Check sheet for the modelled part. Datum: model origin and axes. Units: mm. Face numbers are marked on the shaded views. A direction names the side the tool comes from. Give positions to 0.01 mm unless a question says otherwise; leave off trailing zeros. Write each loop counter-clockwise with the first axis right and the second up, starting at its lowest first coordinate (ties: lowest second). Pieces come first, ordered by that corner, then holes. Notation, with made-up numbers: (-2.5, 81) - (20.5, 81) arc R7 ccw to (20.5, 85) - close; hole circle Ø4 at (-38, 35.25). An arc over 180 degrees is marked (long way). Return JSON: item names as keys, results as strings. Group by question number.
```python
from build123d import *

# Parameters (mm, degrees)
SKETCH1_R           = 15.875
BOSS_EXTRUDE1_DEPTH = 2.54
SKETCH2_R           = 9.525
BOSS_EXTRUDE2_DEPTH = 2.54
SKETCH3_R           = 7.62
CUT_EXTRUDE1_DEPTH  = 3.81
CUT_EXTRUDE2_REACH  = 25.018
SKETCH4_R           = 5.842
CUT_EXTRUDE3_REACH  = 24.594
SKETCH5_R           = 1.7


with BuildPart() as part:
    # Sketch1 → Boss-Extrude1 (new body)
    with BuildSketch(Plane(origin=(0, 0, 0), x_dir=(1, 0, 0), z_dir=(0, 1, 0))):
        with Locations(Location((0, 0, 0), (0, 0, 270))):
            Circle(SKETCH1_R)
    extrude(amount=BOSS_EXTRUDE1_DEPTH)

    # Sketch2 → Boss-Extrude2 (add)
    with BuildSketch(Plane(origin=(0, 2.54, 0), x_dir=(1, 0, 0), z_dir=(0, 1, 0))):
        with Locations(Location((0, 0, 0), (0, 0, 270))):
            Circle(SKETCH2_R)
    extrude(amount=BOSS_EXTRUDE2_DEPTH)

    # Sketch3 → Cut-Extrude1 (cut)
    with BuildSketch(Plane.XZ):
        with Locations(Location((0, 0, 0), (0, 0, 270))):
            Circle(SKETCH3_R)
    extrude(amount=-CUT_EXTRUDE1_DEPTH, mode=Mode.SUBTRACT)

    # Sketch4 → Cut-Extrude2 (cut, up to next)
    with BuildSketch(Plane(origin=(0, 5.08, 0), x_dir=(1, 0, 0), z_dir=(0, 1, 0)), mode=Mode.PRIVATE) as cut_extrude2_sk1:
        with Locations(Location((0, 0, 0), (0, 0, 270))):
            Circle(SKETCH4_R)
    cut_extrude2_tool1 = extrude(cut_extrude2_sk1.sketch, amount=-CUT_EXTRUDE2_REACH, mode=Mode.PRIVATE) & part.part
    add(cut_extrude2_tool1.solids().sort_by_distance((0, 5.08, 0))[0], mode=Mode.SUBTRACT)

    # Sketch5 → Cut-Extrude3 (cut, up to next)
    with BuildSketch(Plane(origin=(0, 2.54, 0), x_dir=(1, 0, 0), z_dir=(0, 1, 0)), mode=Mode.PRIVATE) as cut_extrude3_sk1:
        with Locations(Location((0, 12.7, 0), (0, 0, 270))):
            Circle(SKETCH5_R)
    cut_extrude3_tool1 = extrude(cut_extrude3_sk1.sketch, amount=-CUT_EXTRUDE3_REACH, mode=Mode.PRIVATE) & part.part
    # Sketch5 → Cut-Extrude3 (cut, up to next)
    with BuildSketch(Plane(origin=(0, 2.54, 0), x_dir=(1, 0, 0), z_dir=(0, 1, 0)), mode=Mode.PRIVATE) as cut_extrude3_sk2:
        with Locations(Location((12.7, 0, 0), (0, 0, 270))):
            Circle(SKETCH5_R)
    cut_extrude3_tool2 = extrude(cut_extrude3_sk2.sketch, amount=-CUT_EXTRUDE3_REACH, mode=Mode.PRIVATE) & part.part
    # Sketch5 → Cut-Extrude3 (cut, up to next)
    with BuildSketch(Plane(origin=(0, 2.54, 0), x_dir=(1, 0, 0), z_dir=(0, 1, 0)), mode=Mode.PRIVATE) as cut_extrude3_sk3:
        with Locations(Location((0, -12.7, 0), (0, 0, 270))):
            Circle(SKETCH5_R)
    cut_extrude3_tool3 = extrude(cut_extrude3_sk3.sketch, amount=-CUT_EXTRUDE3_REACH, mode=Mode.PRIVATE) & part.part
    # Sketch5 → Cut-Extrude3 (cut, up to next)
    with BuildSketch(Plane(origin=(0, 2.54, 0), x_dir=(1, 0, 0), z_dir=(0, 1, 0)), mode=Mode.PRIVATE) as cut_extrude3_sk4:
        with Locations(Location((-12.7, 0, 0), (0, 0, 270))):
            Circle(SKETCH5_R)
    cut_extrude3_tool4 = extrude(cut_extrude3_sk4.sketch, amount=-CUT_EXTRUDE3_REACH, mode=Mode.PRIVATE) & part.part
    add(cut_extrude3_tool1.solids().sort_by_distance((0, 2.54, -12.7))[0], mode=Mode.SUBTRACT)
    add(cut_extrude3_tool2.solids().sort_by_distance((12.7, 2.54, 0))[0], mode=Mode.SUBTRACT)
    add(cut_extrude3_tool3.solids().sort_by_distance((0, 2.54, 12.7))[0], mode=Mode.SUBTRACT)
    add(cut_extrude3_tool4.solids().sort_by_distance((-12.7, 2.54, 0))[0], mode=Mode.SUBTRACT)


solid = part.part
```
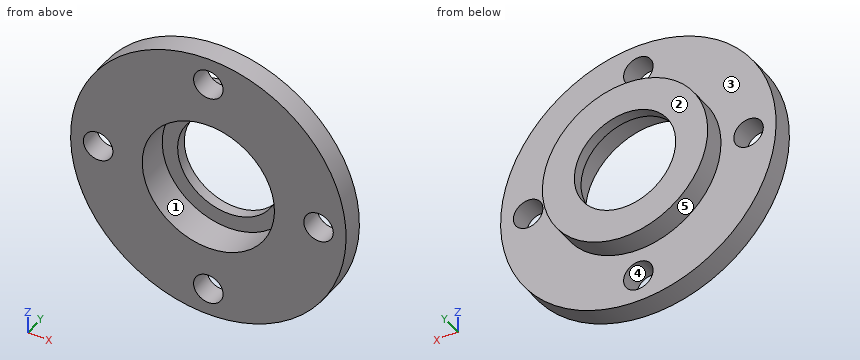
Item 1: Depth check by flat-ended pin: pin 1 (5 mm diameter, centred on x = -3, z = -1, fed in from +Y); pin 2 (3 mm diameter, centred on x = 4, y = 1.5, fed in from +Z); pin 3 (3 mm diameter, centred on x = -3.5, z = 11, fed in from +Y); pin 4 (3 mm diameter, centred on x = -6.5, y = 2, fed in from +Z). Enter the tip coordinate at first touch or a pass-through.
Item 2: Access from +Z, -Z, +X, -X, +Y, -Y to the whole of each face (thin tool, end or side, straight path). Record for the marked faces 1 and 2.
Item 3: Section check D-D on z = 0. Record the cut outline in (x, y) (3 decimals), plus the area to 3 significant figures.
Item 4: Section check A-A on x = 12.7. Record the cut outline in (y, z) (3 decimals), plus the area to 3 significant figures.
Item 5: Material ranges on line 1 along X through (y, z) = (1.15, 0) (3 decimals); line 2 along X through (y, z) = (1.85, 12.7) (3 decimals); line 3 along X through (y, z) = (2.8, 0) (3 decimals), recorded low to high. Write a range as from..to.
Item 6: Section check B-B on z = -12.7. Record the cut outline in (x, y) (3 decimals), plus the area to 3 significant figures.
Item 7: Section check C-C on y = 1.15. Record the cut outline in (x, z) (3 decimals).
Item 8: Mould release check, pull along Z, two halves, no side actions. Record for the marked faces 3, 4 and 5: +Z half, -Z half, draft (parallel to the pull), parting line (faces both ways), or undercut.
Reply:
{
 "1": {"pin 1": "through", "pin 2": "z = 15.68", "pin 3": "y = 2.54", "pin 4": "z = 15.07"},
 "2": {"face 1": "-Y", "face 2": "+Z, -Z, +X, -X, +Y"},
 "3": {"outline": "(-15.875, 0) - (-14.4, 0) - (-14.4, 2.54) - (-15.875, 2.54) - close; (-11, 0) - (-7.62, 0) - (-7.62, 3.81) - (-5.842, 3.81) - (-5.842, 5.08) - (-9.525, 5.08) - (-9.525, 2.54) - (-11, 2.54) - close; (5.842, 3.81) - (7.62, 3.81) - (7.62, 0) - (11, 0) - (11, 2.54) - (9.525, 2.54) - (9.525, 5.08) - (5.842, 5.08) - close; (14.4, 0) - (15.875, 0) - (15.875, 2.54) - (14.4, 2.54) - close", "area": "38.9 mm²"},
 "4": {"outline": "(0, -9.525) - (2.54, -9.525) - (2.54, -1.7) - (0, -1.7) - close; (0, 1.7) - (2.54, 1.7) - (2.54, 9.525) - (0, 9.525) - close", "area": "39.8 mm²"},
 "5": {"line 1": "-15.875..-14.4, -11..-7.62, 7.62..11, 14.4..15.875", "line 2": "-9.525..-1.7, 1.7..9.525", "line 3": "-9.525..-7.62, 7.62..9.525"},
 "6": {"outline": "(-9.525, 0) - (-1.7, 0) - (-1.7, 2.54) - (-9.525, 2.54) - close; (1.7, 0) - (9.525, 0) - (9.525, 2.54) - (1.7, 2.54) - close", "area": "39.8 mm²"},
 "7": {"outline": "circle Ø31.75 at (0, 0); hole circle Ø3.4 at (-12.7, 0); hole circle Ø15.24 at (0, 0); hole circle Ø3.4 at (0, -12.7); hole circle Ø3.4 at (0, 12.7); hole circle Ø3.4 at (12.7, 0)"},
 "8": {"face 3": "draft", "face 4": "undercut", "face 5": "parting line"}
}
